from build123d import *

# Parameters (mm, degrees)
F0_R     = 1.5875
F0_R_2   = 3.175
F1_DEPTH = 3.048


with BuildPart() as f1:
    # F0 (on Front) → F1 (new body)
    with BuildSketch(Plane.XZ):
        with BuildLine():
            ThreePointArc((7.3102929275, 57.069215628), (4.5204850183, 50.3340235372), (-2.2147070725, 47.544215628))
            Line((-2.2147070725, 47.544215628), (-2.2147070725, 22.3989884319))
            ThreePointArc((-2.2147070725, 22.3989884319), (8.2818372765, 18.4335720405), (13.5345178126, 8.5183656578))
            Line((13.5345178126, 8.5183656578), (7.2348278586, 58.2658419636))
            ThreePointArc((7.2348278586, 58.2658419636), (7.2914079389, 57.6687174136), (7.3102929275, 57.069215628))
        make_face()
        with BuildLine():
            Line((-2.2147070725, 22.3989884319), (-2.2147070725, 47.544215628))
            ThreePointArc((-2.2147070725, 47.544215628), (-9.3604572377, 50.7712890187), (-11.6642420035, 58.2658419636))
            Line((-11.6642420035, 58.2658419636), (-17.9639319576, 8.5183656578))
            ThreePointArc((-17.9639319576, 8.5183656578), (-12.7112514214, 18.4335720405), (-2.2147070725, 22.3989884319))
        make_face()
        with Locations((-6.5460577607, 42.0841127634)):
            Circle(F0_R, mode=Mode.SUBTRACT)
        with BuildLine():
            ThreePointArc((-11.6642420035, 58.2658419636), (-9.3604572377, 50.7712890187), (-2.2147070725, 47.544215628))
            ThreePointArc((-2.2147070725, 47.544215628), (4.5204850183, 50.3340235372), (7.3102929275, 57.069215628))
            ThreePointArc((7.3102929275, 57.069215628), (7.2914079389, 57.6687174136), (7.2348278586, 58.2658419636))
            ThreePointArc((7.2348278586, 58.2658419636), (-2.2147070725, 66.594215628), (-11.6642420035, 58.2658419636))
        make_face()
        with Locations((-2.0584128797, 57.1364536881)):
            Circle(F0_R_2, mode=Mode.SUBTRACT)
        with BuildLine():
            ThreePointArc((13.5345178126, 8.5183656578), (8.2818372765, 18.4335720405), (-2.2147070725, 22.3989884319))
            Line((-2.2147070725, 22.3989884319), (-2.2147070725, 9.6537737107))
            ThreePointArc((-2.2147070725, 9.6537737107), (-0.0192566722, 8.6975480096), (0.8837937295, 6.4796954393))
            ThreePointArc((0.8837937295, 6.4796954393), (0.0092186443, 4.2913923956), (-2.132691443, 3.3086549083))
            Line((-2.132691443, 3.3086549083), (-2.132691443, -9.3507997065))
            ThreePointArc((-2.132691443, -9.3507997065), (8.4566239022, -5.2292375181), (13.5784544993, 4.9141211804))
            Line((13.5784544993, 4.9141211804), (13.6405138302, 5.7317794152))
            ThreePointArc((13.6405138302, 5.7317794152), (13.6553473829, 6.1277604865), (13.6602929275, 6.5239884319))
            ThreePointArc((13.6602929275, 6.5239884319), (13.6288179464, 7.5231580745), (13.5345178126, 8.5183656578))
        make_face()
        with BuildLine():
            Line((-2.2147070725, 9.6537737107), (-2.2147070725, 22.3989884319))
            ThreePointArc((-2.2147070725, 22.3989884319), (-12.7112514214, 18.4335720405), (-17.9639319576, 8.5183656578))
            ThreePointArc((-17.9639319576, 8.5183656578), (-18.0842931558, 6.9385515062), (-18.0465791747, 5.3546079379))
            ThreePointArc((-18.0465791747, 5.3546079379), (-12.9885990445, -5.1352944267), (-2.132691443, -9.3507997065))
            Line((-2.132691443, -9.3507997065), (-2.132691443, 3.3086549083))
            ThreePointArc((-2.132691443, 3.3086549083), (-5.4659410707, 6.4386595058), (-2.2147070725, 9.6537737107))
        make_face()
        with BuildLine():
            ThreePointArc((-2.132691443, -9.3507997065), (-12.9885990445, -5.1352944267), (-18.0465791747, 5.3546079379))
            Line((-18.0465791747, 5.3546079379), (-13.3630327903, -58.0544430316))
            ThreePointArc((-13.3630327903, -58.0544430316), (-10.3772327356, -49.5931738227), (-2.132691443, -46.0526064293))
            Line((-2.132691443, -46.0526064293), (-2.132691443, -9.3507997065))
        make_face()
        with BuildLine():
            ThreePointArc((13.5784544993, 4.9141211804), (8.4566239022, -5.2292375181), (-2.132691443, -9.3507997065))
            Line((-2.132691443, -9.3507997065), (-2.132691443, -46.0526064293))
            ThreePointArc((-2.132691443, -46.0526064293), (5.5920407008, -49.2298811623), (8.9582909491, -56.8741548811))
            Line((8.9582909491, -56.8741548811), (36.0931763244, -56.8741548811))
            ThreePointArc((36.0931763244, -56.8741548811), (39.3418040246, -53.517952967), (43.9155275845, -52.5699413526))
            Line((43.9155275845, -52.5699413526), (17.2323900006, -50.0469673747))
            ThreePointArc((17.2323900006, -50.0469673747), (11.9020918829, -47.2560690917), (10.0533689663, -41.530388798))
            Line((10.0533689663, -41.530388798), (13.5784544993, 4.9141211804))
        make_face()
        with BuildLine():
            ThreePointArc((13.5784544993, 4.9141211804), (13.6147644778, 5.322549528), (13.6405138302, 5.7317794152))
            Line((13.6405138302, 5.7317794152), (13.5784544993, 4.9141211804))
        make_face()
        with BuildLine():
            ThreePointArc((-2.132691443, -46.0526064293), (-10.3772327356, -49.5931738227), (-13.3630327903, -58.0544430316))
            ThreePointArc((-13.3630327903, -58.0544430316), (-9.8225389669, -65.4214900969), (-2.2147070725, -68.4096957193))
            ThreePointArc((-2.2147070725, -68.4096957193), (5.6898240232, -65.1355317353), (8.9639880072, -57.2310006396))
            ThreePointArc((8.9639880072, -57.2310006396), (8.9625636519, -57.0525550234), (8.9582909491, -56.8741548811))
            ThreePointArc((8.9582909491, -56.8741548811), (5.5920407008, -49.2298811623), (-2.132691443, -46.0526064293))
        make_face()
        with Locations((-2.2147070725, -57.2310006396)):
            Circle(F0_R_2, mode=Mode.SUBTRACT)
        with BuildLine():
            ThreePointArc((8.9639880072, -57.2310006396), (5.6898240232, -65.1355317353), (-2.2147070725, -68.4096957193))
            Line((-2.2147070725, -68.4096957193), (43.1683447589, -68.4096957193))
            ThreePointArc((43.1683447589, -68.4096957193), (36.4021288518, -64.6221630142), (36.0931763244, -56.8741548811))
            Line((36.0931763244, -56.8741548811), (8.9582909491, -56.8741548811))
            ThreePointArc((8.9582909491, -56.8741548811), (8.9625636519, -57.0525550234), (8.9639880072, -57.2310006396))
        make_face()
        with BuildLine():
            ThreePointArc((36.0931763244, -56.8741548811), (36.4021288518, -64.6221630142), (43.1683447589, -68.4096957193))
            ThreePointArc((43.1683447589, -68.4096957193), (48.7810048346, -66.084855795), (51.1058447589, -60.4721957193))
            ThreePointArc((51.1058447589, -60.4721957193), (49.0392335301, -55.1302324766), (43.9155275845, -52.5699413526))
            ThreePointArc((43.9155275845, -52.5699413526), (39.3418040246, -53.517952967), (36.0931763244, -56.8741548811))
        make_face()
        with Locations((43.4331535689, -60.4018158402)):
            Circle(F0_R_2, mode=Mode.SUBTRACT)
    extrude(amount=F1_DEPTH)


solid = f1.part
Verification items for the finished model (mm, model axes). A direction names the side the tool comes from. Coordinates: 2 decimals unless noted, no trailing zeros. Loops run counter-clockwise (first coordinate to the right, second up) from the corner with the lowest first, then second, coordinate; pieces in that order, holes last. Notation, with made-up numbers: (57.25, -19.75) -> (74.25, -19.75) arc R32 cw to (74.25, 12.25) -> close; hole circle Ø8 at (26, 49). An arc over 180 degrees is marked (long way). Answer as a JSON object with one key per item and string values. Group by question number.
Item 1: Scan lines: probe 1 along Z at (x, y) = (-2, -1.3); probe 2 along X at (y, z) = (-1.8, 9); probe 3 along Z at (x, y) = (43, -2.55). Record each from-to range of solid material in increasing order.
Item 2: Tool access check on faces 5 (the cylindrical face through (-2.022, -1.503, 66.592)), 6 (the cylindrical face through (11.958, -1.503, -47.322)). Record the directions out of +Z, -Z, +X, -X, +Y, -Y that give a thin tool (end or side, any length) a straight path to the whole face; none if there is none.
Item 3: Sectioned sample at C-C on z = -2.5. Record the boundary of the cut face in (x, y).
Item 4: Sectioned sample at D-D on x = 34.5. Record the boundary of the cut face in (y, z).
Item 5: Sectioned sample at B-B on y = -1.05. State how many separate pieces and enclosed holes the cut face has, plus the area to 3 significant figures.
Item 6: Depth check by flat-ended pin: pin 1 (1 mm diameter, centred on y = -2, z = 3, fed in from -X); pin 2 (1 mm diameter, centred on y = -1, z = 22, fed in from -X); pin 3 (10 mm diameter, centred on x = -2.06, z = 57.14, fed in from -Y); pin 4 (1.5 mm diameter, centred on y = -2, z = -28, fed in from +X). Enter the tip coordinate at first touch or a pass-through.
Item 7: Mould release check, pull along X, two halves, no side actions. Record for faces 1 (the cylindrical face through (-6.89, -1.503, 40.534)), 2 (the flat face through (30.761, -1.503, -51.326)), 3 (the flat face through (1, 0, -15)), 4 (the cylindrical face through (-0.352, -1.503, 59.814)): +X half, -X half, draft (parallel to the pull), parting line (faces both ways), or undercut.
Item 8: Sectioned sample at A-A on x = -0.5. Record the boundary of the cut face in (y, z).
Evaluation:
{
 "1": {"probe 1": "z = -68.41 to -60.4, -54.06 to 3.32, 9.64 to 53.96, 60.31 to 66.59", "probe 2": "x = -17.9 to -4.22, -0.36 to 13.47", "probe 3": "z = -68.41 to -63.55, -57.26 to -52.48"},
 "2": {"face 5": "+Z, +Y, -Y", "face 6": "+X, +Y, -Y"},
 "3": {"outline": "(-17.47, -3.05) -> (13.02, -3.05) -> (13.02, 0) -> (-17.47, 0) -> close"},
 "4": {"outline": "(-3.05, -68.41) -> (0, -68.41) -> (0, -51.68) -> (-3.05, -51.68) -> close"},
 "5": {"separate pieces": "1", "enclosed holes": "5", "area": "3,960 mm²"},
 "6": {"pin 1": "stops at x = -17.91", "pin 2": "stops at x = -16.32", "pin 3": "stops at y = -3.05", "pin 4": "stops at x = 11.14"},
 "7": {"face 1": "undercut", "face 2": "+X half", "face 3": "draft", "face 4": "undercut"},
 "8": {"outline": "(-3.05, -68.41) -> (0, -68.41) -> (0, -59.9) -> (-3.05, -59.9) -> close; (-3.05, -54.56) -> (0, -54.56) -> (0, 3.86) -> (-3.05, 3.86) -> close; (-3.05, 9.1) -> (0, 9.1) -> (0, 54.37) -> (-3.05, 54.37) -> close; (-3.05, 59.9) -> (0, 59.9) -> (0, 66.44) -> (-3.05, 66.44) -> close"}
}
